Check sheet for the drawn part. Datum: minimum x, y, z corner. Units: mm. Coordinates: 2 decimals unless noted, no trailing zeros. Write each loop counter-clockwise with the first axis right and the second up, starting at its lowest first coordinate (ties: lowest second). Pieces come first, ordered by that corner, then holes. Notation, with made-up numbers: (42, 4) -> (70, 4) arc R31 ccw to (70, 32) -> close; hole circle Ø9 at (-32, 32). An arc over 180 degrees is marked (long way). Write each question's results on one line, items separated by ' | '. Start each with the question number.
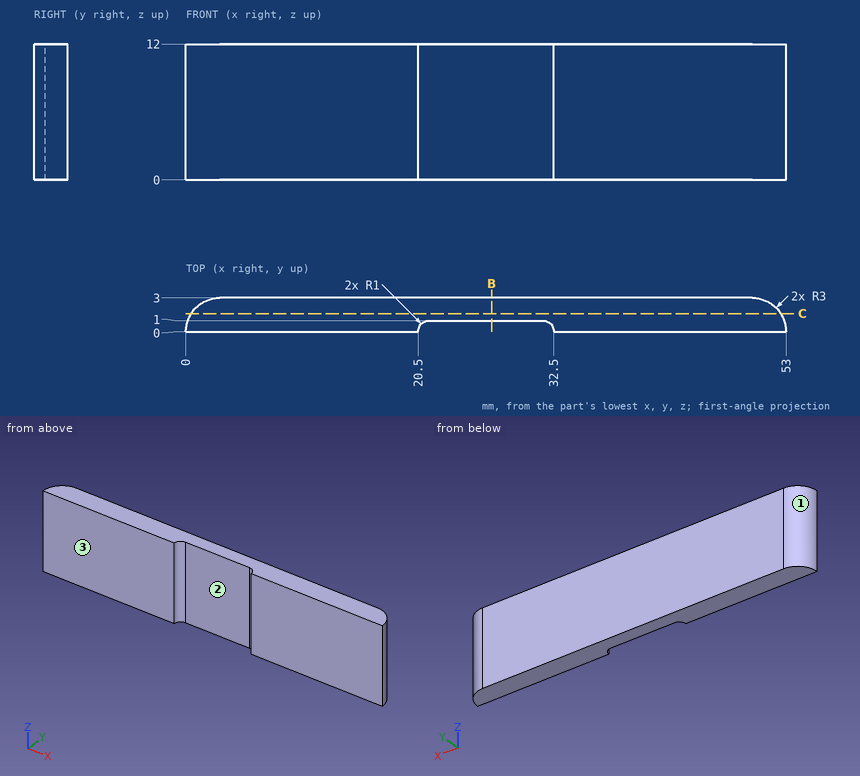
1. Mould release check, pull along X, two halves, no side actions. Record for the marked faces 1, 2 and 3: +X half, -X half, draft (parallel to the pull), parting line (faces both ways), or undercut.
2. Material ranges on probe 1 along Y at (x, z) = (29.5, 7.75); probe 2 along X at (y, z) = (0.45, 2); probe 3 along X at (y, z) = (0.7, 9), recorded low to high. Write a range as from..to.
3. Depth check by flat-ended pin: pin 1 Ø5 at (x, z) = (25, 6) entering from -Y. Enter the tip coordinate at first touch or a pass-through.
4. Sectioned sample at B-B on x = 27. Record the cut outline in (y, z), plus the area to 3 significant figures.
5. Sectioned sample at C-C on y = 1.6. Record the cut outline in (x, z), plus the area to 3 significant figures.
Computed values:
1) face 1: -X half | face 2: undercut | face 3: draft
2) probe 1: y = 1..3 | probe 2: x = 0.03..20.61, 32.39..52.97 | probe 3: x = 0.08..20.79, 32.21..52.92
3) pin 1: stops at y = 1
4) outline: (1, 0) -> (3, 0) -> (3, 12) -> (1, 12) -> close | area: 24.0 mm^2
5) outline: (0.46, 0) -> (52.54, 0) -> (52.54, 12) -> (0.46, 12) -> close | area: 625 mm^2
